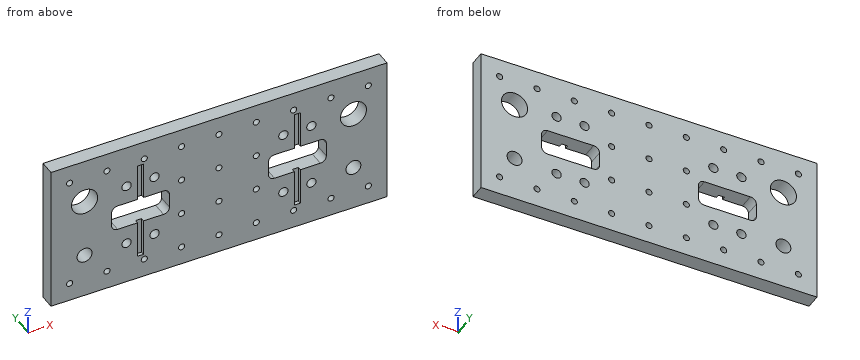
```python
from build123d import *

# Parameters (mm, degrees)
SKETCH1_W           = 180
SKETCH1_H           = 80
BOSS_EXTRUDE1_DEPTH = 8
SKETCH2_R           = 4
SKETCH2_R_2         = 7
SKETCH2_W           = 31
SKETCH2_H           = 14
CUT_EXTRUDE1_DEPTH  = 30
FILLET1_R           = 3.2
SKETCH5_R           = 1.65
CUT_EXTRUDE4_DEPTH  = 8
SKETCH3_W           = 3.2
SKETCH3_H           = 20
CUT_EXTRUDE5_DEPTH  = 2
SKETCH7_R           = 2.5
CUT_EXTRUDE6_DEPTH  = 198.139544486


with BuildPart() as part:
    # Sketch1 → Boss-Extrude1 (new body)
    with BuildSketch(Plane(origin=(0, 0, 0), x_dir=(1, 0, 0), z_dir=(0, 1, 0))):
        with Locations((90, -40)):
            Rectangle(SKETCH1_W, SKETCH1_H)
    extrude(amount=BOSS_EXTRUDE1_DEPTH)

    # Sketch2 → Cut-Extrude1 (cut)
    with BuildSketch(Plane(origin=(0, 8, 0), x_dir=(1, 0, 0), z_dir=(0, 1, 0))):
        with Locations(Location((18, -24, 0), (0, 0, 270))):
            Circle(SKETCH2_R)
        with Locations(Location((162, -24, 0), (0, 0, 270))):
            Circle(SKETCH2_R)
        with Locations(Location((18, -56, 0), (0, 0, 270))):
            Circle(SKETCH2_R_2)
        with Locations(Location((162, -56, 0), (0, 0, 270))):
            Circle(SKETCH2_R_2)
        with Locations((132, -40)):
            Rectangle(SKETCH2_W, SKETCH2_H)
        with Locations((48, -40)):
            Rectangle(SKETCH2_W, SKETCH2_H)
    extrude(amount=-CUT_EXTRUDE1_DEPTH, mode=Mode.SUBTRACT)

    # Fillet1
    fillet1_edges = [part.edges().sort_by_distance(p)[0] for p in [
        (32.5, 4, 47),
        (32.5, 4, 33),
        (63.5, 4, 33),
        (63.5, 4, 47),
        (116.5, 4, 33),
        (147.5, 4, 33),
        (147.5, 4, 47),
        (116.5, 4, 47),
    ]]
    fillet(fillet1_edges, radius=FILLET1_R)

    # Sketch5 → Cut-Extrude4 (cut)
    with BuildSketch(Plane(origin=(0, 8, 0), x_dir=(1, 0, 0), z_dir=(0, 1, 0))):
        with Locations(Location((90, -10, 0), (0, 0, 270))):
            Circle(SKETCH5_R)
        with Locations(Location((70, -10, 0), (0, 0, 270))):
            Circle(SKETCH5_R)
        with Locations(Location((50, -10, 0), (0, 0, 270))):
            Circle(SKETCH5_R)
        with Locations(Location((30, -10, 0), (0, 0, 270))):
            Circle(SKETCH5_R)
        with Locations(Location((10, -10, 0), (0, 0, 270))):
            Circle(SKETCH5_R)
        with Locations(Location((170, -10, 0), (0, 0, 90))):
            Circle(SKETCH5_R)
        with Locations(Location((150, -10, 0), (0, 0, 90))):
            Circle(SKETCH5_R)
        with Locations(Location((130, -10, 0), (0, 0, 90))):
            Circle(SKETCH5_R)
        with Locations(Location((110, -10, 0), (0, 0, 90))):
            Circle(SKETCH5_R)
        with Locations(Location((170, -70, 0), (0, 0, 270))):
            Circle(SKETCH5_R)
        with Locations(Location((150, -70, 0), (0, 0, 270))):
            Circle(SKETCH5_R)
        with Locations(Location((130, -70, 0), (0, 0, 270))):
            Circle(SKETCH5_R)
        with Locations(Location((110, -70, 0), (0, 0, 270))):
            Circle(SKETCH5_R)
        with Locations(Location((90, -70, 0), (0, 0, 90))):
            Circle(SKETCH5_R)
        with Locations(Location((70, -70, 0), (0, 0, 90))):
            Circle(SKETCH5_R)
        with Locations(Location((50, -70, 0), (0, 0, 90))):
            Circle(SKETCH5_R)
        with Locations(Location((30, -70, 0), (0, 0, 90))):
            Circle(SKETCH5_R)
        with Locations(Location((10, -70, 0), (0, 0, 90))):
            Circle(SKETCH5_R)
        with Locations(Location((90, -30, 0), (0, 0, 270))):
            Circle(SKETCH5_R)
        with Locations(Location((90, -50, 0), (0, 0, 90))):
            Circle(SKETCH5_R)
        with Locations(Location((70, -50, 0), (0, 0, 270))):
            Circle(SKETCH5_R)
        with Locations(Location((70, -30, 0), (0, 0, 90))):
            Circle(SKETCH5_R)
        with Locations(Location((110, -50, 0), (0, 0, 270))):
            Circle(SKETCH5_R)
        with Locations(Location((110, -30, 0), (0, 0, 90))):
            Circle(SKETCH5_R)
    extrude(amount=-CUT_EXTRUDE4_DEPTH, mode=Mode.SUBTRACT)

    # Sketch3 → Cut-Extrude5 (cut)
    with BuildSketch(Plane.XZ):
        with Locations((48, 23)):
            Rectangle(SKETCH3_W, SKETCH3_H)
        with Locations((48, 57)):
            Rectangle(SKETCH3_W, SKETCH3_H)
        with Locations((132, 23)):
            Rectangle(SKETCH3_W, SKETCH3_H)
        with Locations((132, 57)):
            Rectangle(SKETCH3_W, SKETCH3_H)
    extrude(amount=-CUT_EXTRUDE5_DEPTH, mode=Mode.SUBTRACT)

    # Sketch7 → Cut-Extrude6 (cut, through all)
    with BuildSketch(Plane.XZ):
        with Locations(Location((40.5, 57, 0), (0, 0, 270))):
            Circle(SKETCH7_R)
        with Locations(Location((55.5, 57, 0), (0, 0, 90))):
            Circle(SKETCH7_R)
        with Locations(Location((55.5, 23, 0), (0, 0, 270))):
            Circle(SKETCH7_R)
        with Locations(Location((40.5, 23, 0), (0, 0, 90))):
            Circle(SKETCH7_R)
        with Locations(Location((124.5, 23, 0), (0, 0, 90))):
            Circle(SKETCH7_R)
        with Locations(Location((139.5, 23, 0), (0, 0, 270))):
            Circle(SKETCH7_R)
        with Locations(Location((124.5, 57, 0), (0, 0, 270))):
            Circle(SKETCH7_R)
        with Locations(Location((139.5, 57, 0), (0, 0, 90))):
            Circle(SKETCH7_R)
    extrude(amount=-CUT_EXTRUDE6_DEPTH, mode=Mode.SUBTRACT)


solid = part.part
```
Source: CAD feature listing. Evaluate the final solid. Frame: model axes, mm. Coordinates: 2 decimals unless noted, no trailing zeros. Write each loop counter-clockwise with the first axis right and the second up, starting at its lowest first coordinate (ties: lowest second). Pieces come first, ordered by that corner, then holes. Notation, with made-up numbers: (-16, 59.5) -> (13, 59.5) arc R18 cw to (13, 86.5) -> close; hole circle Ø5 at (52, -14). An arc over 180 degrees is marked (long way). Return JSON: item names as keys, results as strings. Group by question number.
1) Section query B-B, the plane y = 3.75. State how many separate pieces and enclosed holes the cut face has, plus the area to 3 significant figures.
2) Ray query, line 1 along Z through (x, y) = (110, 3); line 2 along Z through (x, y) = (170, 4.25); line 3 along X through (y, z) = (4, 60). Return the intervals inside material, ascending.
3) Section query A-A, the plane x = 55.5. Return loops of the section in (y, z).
4) Contact query for a flat-ended pin moving along its axis: P1, Ø4, axis at x = 131, y = 5.5, coming from the -Z side. Output: stop coordinate, or through.
From the geometry:
{
 "1": {"separate pieces": "1", "enclosed holes": "38", "area": "12,800 mm²"},
 "2": {"line 1": "0 to 8.35, 11.65 to 28.35, 31.65 to 48.35, 51.65 to 68.35, 71.65 to 80", "line 2": "0 to 8.35, 11.65 to 68.35, 71.65 to 80", "line 3": "0 to 12.26, 23.74 to 156.26, 167.74 to 180"},
 "3": {"outline": "(0, 0) -> (8, 0) -> (8, 20.5) -> (0, 20.5) -> close; (0, 25.5) -> (8, 25.5) -> (8, 33) -> (0, 33) -> close; (0, 47) -> (8, 47) -> (8, 54.5) -> (0, 54.5) -> close; (0, 59.5) -> (8, 59.5) -> (8, 80) -> (0, 80) -> close"},
 "4": {"P1": "z = 0"}
}
